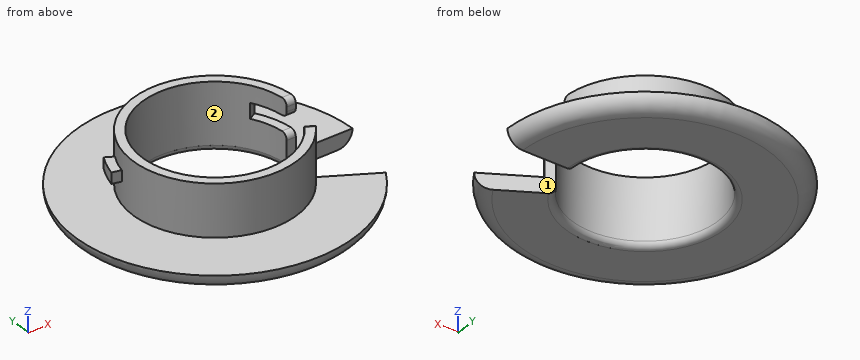
from build123d import *

# Parameters (mm, degrees)
F3_DEPTH      = 17.001
F3_DEPTH_BACK = 25
F6_DEPTH      = 2.5
F7_R          = 2
F8_DEPTH      = 1.8


with BuildPart() as f1:
    # F0 (on Front) → F1 (revolve)
    with BuildSketch(Plane.XZ):
        with BuildLine():
            Line((-23.8, 17), (-26.8, 17))
            Line((-26.8, 17), (-26.8, 0))
            Line((-26.8, 0), (-45.6279513852, 0))
            ThreePointArc((-45.6279513852, 0), (-44.1634852911, -3.5355339059), (-40.6279513852, -5))
            Line((-40.6279513852, -5), (-25.8, -5))
            ThreePointArc((-25.8, -5), (-24.3857864376, -4.4142135624), (-23.8, -3))
            Line((-23.8, -3), (-23.8, 17))
        make_face()
    revolve(axis=Axis((0, 0, 7.2955568321), (0, 0, 1)))

    # F2 (on Top) → F3 (cut, two sides)
    with BuildSketch(Plane.XY) as f3_sk:
        Polygon((53.3640757203, 0), (0, 0), (46.3265438035, -26.7466425355), align=None)
    extrude(amount=F3_DEPTH, mode=Mode.SUBTRACT)
    extrude(f3_sk.sketch, amount=-F3_DEPTH_BACK, mode=Mode.SUBTRACT)

    # F5 (on offset) → F6 (cut, symmetric)
    with BuildSketch(Plane.XY.offset(9)):
        Polygon((26.6670817875, 15.3962468485), (0, 0), (30.5216945708, 0), align=None)
    extrude(amount=F6_DEPTH, both=True, mode=Mode.SUBTRACT)

    # F7
    f7_edges = [f1.edges().sort_by_distance(p)[0] for p in [
        (21.910443, -12.65, 17),
        (25.3, 0, 17),
        (25.3, 0, 11.5),
        (25.3, 0, 6.5),
    ]]
    fillet(f7_edges, radius=F7_R)

    # F5 (on offset) → F8 (join, symmetric)
    with BuildSketch(Plane.XY.offset(9)):
        with BuildLine():
            Line((-21.9827251313, 12.2826441446), (-26.0146328451, 14.535435251))
            ThreePointArc((-26.0146328451, 14.535435251), (-27.6893290703, 11.0154916202), (-28.8902531983, 7.3070698737))
            Line((-28.8902531983, 7.3070698737), (-23.0896898866, 5.8399618793))
            Line((-23.0896898866, 5.8399618793), (-21.9827251313, 12.2826441446))
        make_face()
    extrude(amount=F8_DEPTH, both=True)


solid = f1.part
Work out the finished part from the listing and answer in its coordinate system (mm). Face numbers are marked on the shaded views. A direction names the side the tool comes from. Give positions to 0.01 mm unless a question says otherwise; leave off trailing zeros. Order: outer loops, then holes, each group sorted by start corner. A loop starts at its lowest first (then second) coordinate and runs counter-clockwise, first axis right, second up. Notation, with made-up numbers: (44, 14) -> (53, 14) arc R18 cw to (53, 35) -> close; hole circle Ø5 at (40.25, 4). An arc over 180 degrees is marked (long way). Answer as a JSON object with one key per item and string values. Group by question number.
1. Consider line 1 along Y through (x, z) = (0, 8); line 2 along Z through (x, y) = (28, 29.5); line 3 along Y through (x, z) = (3, -2.25). Determine where each line is inside the solid, lowest interval first. Write a range as [from, to].
2. Section A-A on x = 0 is taken. Determine the outline of the cut face in (y, z).
3. Flat-ended cylindrical pins translate along their axes: pin 1 Ø8 at (x, z) = (-1, 8) entering from +Y; pin 2 Ø12 at (y, z) = (-28, -0.5) entering from +X; pin 3 Ø5 at (x, z) = (-18, 8.5) entering from -Y. Find the tip coordinate at first contact, or state that the pin passes through.
4. A tool of negligible diameter and unlimited length cuts with its end or side. For the marked faces 1 and 2, from which of +Z, -Z, +X, -X, +Y, -Y can it reach the whole face along a straight path? Write none if from no direction.
Result sheet:
{
 "1": {"line 1": "y = [-26.8, -23.8], [23.8, 26.8]", "line 2": "z = [-5, 0]", "line 3": "y = [-44.99, -23.61], [23.61, 44.99]"},
 "2": {"outline": "(-45.63, 0) arc R5 ccw to (-40.63, -5) -> (-25.8, -5) arc R2 ccw to (-23.8, -3) -> (-23.8, 17) -> (-26.8, 17) -> (-26.8, 0) -> close; (23.8, -3) arc R2 ccw to (25.8, -5) -> (40.63, -5) arc R5 ccw to (45.63, 0) -> (26.8, 0) -> (26.8, 17) -> (23.8, 17) -> close"},
 "3": {"pin 1": "stops at y = 26.8", "pin 2": "stops at x = 39.51", "pin 3": "stops at y = -21.86"},
 "4": {"face 1": "+Z, -Z, +X", "face 2": "+Z, -Z"}
}
